```python
from build123d import *


with BuildPart() as part:
    # Sketch1 → Revolve1 (revolve)
    with BuildSketch(Plane.XY):
        Polygon((220, 45), (220, 60), (-180, 60), (-180, 12), (-220, 12), (-220, 0), (-160, 0), (-160, 55), (200, 55), (200, 45), align=None)
    revolve(axis=Axis((-220, 0, 0), (1, 0, 0)))

    # Sketch2 → Ball (revolve)
    with BuildSketch(Plane.XY):
        with BuildLine():
            Line((-240.493320132, 0), (-212.973320132, 0))
            ThreePointArc((-212.973320132, 0), (-226.733320132, 13.76), (-240.493320132, 0))
        make_face()
    revolve(axis=Axis((-240.493320132, 0, 0), (1, 0, 0)))


solid = part.part
```
Design review of the part built by this model. Coordinates are the model's own, in mm. A direction names the side the tool comes from. Give positions to 0.01 mm unless a question says otherwise; leave off trailing zeros. Write each loop counter-clockwise with the first axis right and the second up, starting at its lowest first coordinate (ties: lowest second). Pieces come first, ordered by that corner, then holes.
(1) Wall thickness on line 1 along Y through (x, z) = (130, -1); line 2 along X through (y, z) = (-27, -41); line 3 along Z through (x, y) = (207, 0): over which ranges is each line inside the solid? List them lowest first.
Checked values:
line 1: y = -59.99 to -54.99, 54.99 to 59.99
line 2: x = -180 to -160, 200 to 220
line 3: z = -60 to -45, 45 to 60
(2) Add section B-B (x = -18). Give the boundary of the cut face in (y, z), and give its area (3 significant figures).
Checked values:
outline: circle Ø120 at (0, 0); hole circle Ø110 at (0, 0)
area: 1,810 mm2
(3) Tool access review of faces 1 (the face through (210.14, 20.765, -39.923)), 2 (the face through (220, -9, 45)), 3 (the face through (-160, 1, 1)): name each direction out of +Z, -Z, +X, -X, +Y, -Y from which nothing blocks a thin tool from reaching the whole face with its end or side.
Checked values:
face 1: +X
face 2: +Z, -Z, +X, +Y, -Y
face 3: none
(4) Add section A-A (z = 0). Give the boundary of the cut face in (x, y).
Checked values:
outline: (-220, -12) - (-180, -12) - (-180, -60) - (220, -60) - (220, -45) - (200, -45) - (200, -55) - (-160, -55) - (-160, 55) - (200, 55) - (200, 45) - (220, 45) - (220, 60) - (-180, 60) - (-180, 12) - (-220, 12) arc R13.76 ccw (long way) to start
(5) Add section D-D (z = 50). Give the boundary of the cut face in (x, y).
Checked values:
outline: (-180, -33.17) - (220, -33.17) - (220, 33.17) - (-180, 33.17) - close; hole (-160, -22.91) - (200, -22.91) - (200, 22.91) - (-160, 22.91) - close
(6) Mouldability with a two-part tool opening along Y and no side actions: class faces 4 (the face through (17.2, -59.94, 2.64)), 5 (the face through (200, -21, -40)), 6 (the face through (-180, -0.8, -12.5)) as +Y half, -Y half, draft (parallel to the pull), parting line (faces both ways), or undercut.
Checked values:
face 4: parting line
face 5: undercut
face 6: draft
(7) Clearance check with flat-ended pins moving along their axes: pin 1 Ø2 at (x, z) = (119.5, 21) entering from -Y; pin 2 Ø4 at (x, z) = (133, -3.5) entering from -Y; pin 3 Ø10 at (x, y) = (-44, -3) entering from +Z. State where each tip first meets the part, or that it passes through.
Checked values:
pin 1: stops at y = -56.57
pin 2: stops at y = -59.98
pin 3: stops at z = 60
(8) Add section C-C (y = -28). Give the boundary of the cut face in (x, z).
Checked values:
outline: (-180, -53.07) - (220, -53.07) - (220, -35.23) - (200, -35.23) - (200, -47.34) - (-160, -47.34) - (-160, 47.34) - (200, 47.34) - (200, 35.23) - (220, 35.23) - (220, 53.07) - (-180, 53.07) - close
